```python
from build123d import *

# Parameters (mm, degrees)
EXTRUDE_1_DEPTH     = 12
SKETCH_2_R          = 1.5
CUT_EXTRUDE_1_DEPTH = 46.475268004


with BuildPart() as part:
    # 草图1 → 凸台-拉伸1 (new body)
    with BuildSketch(Plane.XY):
        Polygon((40, 0), (-40, 0), (-40, 18), (-25.5, 18), (-25.5, 15), (25.5, 15), (25.5, 18), (40, 18), align=None)
    extrude(amount=EXTRUDE_1_DEPTH)

    # 草图2 → 切除-拉伸1 (cut, through all)
    with BuildSketch(Plane.XZ):
        with Locations(Location((-32.5, 6, 0), (0, 0, 270))):
            Circle(SKETCH_2_R)
        with Locations(Location((32.5, 6, 0), (0, 0, 90))):
            Circle(SKETCH_2_R)
    extrude(amount=-CUT_EXTRUDE_1_DEPTH, mode=Mode.SUBTRACT)


solid = part.part
```
Model file for the job. Use its own axes, mm. A direction names the side the tool comes from. Give positions to 0.01 mm unless a question says otherwise; leave off trailing zeros. Loops run counter-clockwise (first coordinate to the right, second up) from the corner with the lowest first, then second, coordinate; pieces in that order, holes last. Notation, with made-up numbers: (52, -28) - (85, -28) arc R28 cw to (85, 8) - close; hole circle Ø3 at (86, 23.5). An arc over 180 degrees is marked (long way). One line per item, written item: value. Start each with the question number.
1. Slice it at C-C (z = 1.5). List the corners of the cut face in (x, y).
2. Slice it at D-D (x = -18.5). List the corners of the cut face in (y, z), plus the area to 3 significant figures.
3. Slice it at A-A (x = 32.5). List the corners of the cut face in (y, z).
4. Slice it at B-B (z = 6). List the corners of the cut face in (x, y), plus the area to 3 significant figures.
5. Pin check, flat tips, straight feed: pin 1 (6 mm diameter, centred on x = -9, z = 7, fed in from +Y); pin 2 (4 mm diameter, centred on x = -26.5, y = 15, fed in from -Z). Stop position of each tip, or through.
6. Probe L1, parallel to X at y = 11.5, z = 6; L2, parallel to X at y = 16.75, z = 11.75; L3, parallel to Z at x = 32.5, y = 5.75. List the from-to ranges inside material, lowest first. Write a range as from..to.
7. Pull direction X, two halves, no side cores. Call faces 3 (the flat face through (34.3, 18, 5.9)), 4 (the flat face through (40, 9, 6)), 5 (the flat face through (-25.5, 17, 6)), 6 (the flat face through (-40, 9, 6)): pulls with the +X half, pulls with the -X half, needs draft (parallel to the pull), parting line crosses it, or undercut.
8. Which spindle directions (+Z, -Z, +X, -X, +Y, -Y) get a long thin tool onto all of the face, cutting with end or side? Do faces 1 (the flat face through (25.5, 16, 6)), 2 (the flat face through (-34.5, 18, 5.9)). Say none if no direction does.
Solution:
1. outline: (-40, 0) - (40, 0) - (40, 18) - (25.5, 18) - (25.5, 15) - (-25.5, 15) - (-25.5, 18) - (-40, 18) - close
2. outline: (0, 0) - (15, 0) - (15, 12) - (0, 12) - close
2. area: 180 mm^2
3. outline: (0, 0) - (18, 0) - (18, 4.5) - (0, 4.5) - close; (0, 7.5) - (18, 7.5) - (18, 12) - (0, 12) - close
4. outline: (-40, 0) - (-34, 0) - (-34, 18) - (-40, 18) - close; (-31, 0) - (31, 0) - (31, 18) - (25.5, 18) - (25.5, 15) - (-25.5, 15) - (-25.5, 18) - (-31, 18) - close; (34, 0) - (40, 0) - (40, 18) - (34, 18) - close
4. area: 1,180 mm^2
5. pin 1: stops at y = 15
5. pin 2: stops at z = 0
6. L1: x = -40..-34, -31..31, 34..40
6. L2: x = -40..-25.5, 25.5..40
6. L3: z = 0..4.5, 7.5..12
7. face 3: needs draft
7. face 4: pulls with the +X half
7. face 5: undercut
7. face 6: pulls with the -X half
8. face 1: +Z, -Z, +Y
8. face 2: +Z, -Z, +X, -X, +Y
